from build123d import *

# Parameters (mm, degrees)
SKETCH1_R                                        = 2
BOSS_EXTRUDE1_DEPTH                              = 15
CUT_EXTRUDE7_START                               = 15
SKETCH1_3_R                                      = 5
CUT_EXTRUDE7_DEPTH                               = 4
CUT_EXTRUDE2_START                               = -22.5000001
CUT_EXTRUDE2_DEPTH                               = 45.0000001
CUT_EXTRUDE6_DEPTH                               = 30
CBORE_FOR_M3_HEX_HEAD_MACHINE_SCREW3_D           = 3
CBORE_FOR_M3_HEX_HEAD_MACHINE_SCREW3_DEPTH       = 25
CBORE_FOR_M3_HEX_HEAD_MACHINE_SCREW3_CBORE_D     = 6
CBORE_FOR_M3_HEX_HEAD_MACHINE_SCREW3_CBORE_DEPTH = 18
CBORE_FOR_M3_HEX_HEAD_MACHINE_SCREW3_TIP         = 0.901290929
CUT_EXTRUDE4_START                               = 15
SKETCH19_R                                       = 2.15
SKETCH19_R_2                                     = 2.25
CUT_EXTRUDE4_DEPTH                               = 10
CUT_EXTRUDE5_START                               = -5
SKETCH19_2_R                                     = 2.15
SKETCH19_2_R_2                                   = 2.25
CUT_EXTRUDE5_DEPTH                               = 10
BOSS_EXTRUDE3_DEPTH                              = 2.5
CBORE_FOR_M3_SHCS2_D                             = 3
CBORE_FOR_M3_SHCS2_DEPTH                         = 12
CBORE_FOR_M3_SHCS2_CBORE_D                       = 4.3
CBORE_FOR_M3_SHCS2_CBORE_DEPTH                   = 5.2
CBORE_FOR_M3_SHCS3_D                             = 2.5
CBORE_FOR_M3_SHCS3_DEPTH                         = 12
CBORE_FOR_M3_SHCS3_CBORE_D                       = 4.3
CBORE_FOR_M3_SHCS3_CBORE_DEPTH                   = 5.2
FILLET2_R                                        = 5
CUT_EXTRUDE9_START                               = -15
SKETCH1_5_R                                      = 5
CUT_EXTRUDE9_DEPTH                               = 3


# Read off the part's stored shape, not the designer's step: Cut-Extrude2
with BuildPart() as part:
    # Sketch1 → Boss-Extrude1 (new, symmetric)
    with BuildSketch(Plane.XY):
        with BuildLine():
            Line((0, 17.5), (0, -17.5))
            add(Edge.make_bspline(
                [(0, -17.5), (43.884108447, -9.177006937), (123.842028205, -11.029704256), (170, -22.5)],
                knots=[0, 0, 0, 0, 1, 1, 1, 1], degree=3))
            ThreePointArc((170, -22.5), (192.5, 0), (170, 22.5))
            add(Edge.make_bspline(
                [(170, 22.5), (123.842028205, 11.029704256), (43.884108447, 9.177006937), (0, 17.5)],
                knots=[0.933681919, 0.933681919, 0.933681919, 0.933681919, 1.933681919, 1.933681919, 1.933681919, 1.933681919], degree=3))
        make_face()
        with Locations((175.71763899, 11.115691808)):
            Circle(SKETCH1_R, mode=Mode.SUBTRACT)
        with Locations((164.28236101, -11.115691808)):
            Circle(SKETCH1_R, mode=Mode.SUBTRACT)
        with Locations((178.447925774, -4.345405633)):
            Circle(SKETCH1_R, mode=Mode.SUBTRACT)
        with Locations((161.552074226, 4.345405633)):
            Circle(SKETCH1_R, mode=Mode.SUBTRACT)
    extrude(amount=BOSS_EXTRUDE1_DEPTH, both=True)

    # Sketch1<3> → Cut-Extrude7 (cut)
    with BuildSketch(Plane.XY.offset(CUT_EXTRUDE7_START)):
        with Locations((170, 0)):
            Circle(SKETCH1_3_R)
    extrude(amount=-CUT_EXTRUDE7_DEPTH, mode=Mode.SUBTRACT)

    # Cut-Extrude2 outline → Cut-Extrude2 (cut)
    with BuildSketch(Plane(origin=(0, 0, 0), x_dir=(1, 0, 0), z_dir=(0, 1, 0)).offset(CUT_EXTRUDE2_START)):
        Polygon((14.999999991, -15.000000001), (194, -15), (194, 7.185915493), (192.500000099, 7.000000012), align=None)
    extrude(amount=CUT_EXTRUDE2_DEPTH, mode=Mode.SUBTRACT)

    # Sketch20 → Cut-Extrude6 (cut, symmetric)
    with BuildSketch(Plane(origin=(0, 0, 0), x_dir=(1, 0, 0), z_dir=(0, 1, 0))):
        Polygon((15, -9), (15, 9), (160, 9), (160, 8.971830985), align=None)
    extrude(amount=CUT_EXTRUDE6_DEPTH, both=True, mode=Mode.SUBTRACT)

    # CBORE for M3 Hex Head Machine Screw3
    with Locations(Plane(origin=(0, 0, 10), x_dir=(-1, 0, 0), z_dir=(0, 0, 1))):
        with Locations((-175.71763899, -11.115691808), (-161.552074226, -4.345405633), (-164.28236101, 11.115691808), (-178.447925774, 4.345405633)):
            CounterBoreHole(CBORE_FOR_M3_HEX_HEAD_MACHINE_SCREW3_D / 2, CBORE_FOR_M3_HEX_HEAD_MACHINE_SCREW3_CBORE_D / 2, CBORE_FOR_M3_HEX_HEAD_MACHINE_SCREW3_CBORE_DEPTH, depth=CBORE_FOR_M3_HEX_HEAD_MACHINE_SCREW3_DEPTH)
            with Locations((0, 0, -(CBORE_FOR_M3_HEX_HEAD_MACHINE_SCREW3_DEPTH + CBORE_FOR_M3_HEX_HEAD_MACHINE_SCREW3_TIP / 2))):  # 118° drill point
                Cone(0, CBORE_FOR_M3_HEX_HEAD_MACHINE_SCREW3_D / 2, CBORE_FOR_M3_HEX_HEAD_MACHINE_SCREW3_TIP, mode=Mode.SUBTRACT)

    # Sketch19 → Cut-Extrude4 (cut)
    with BuildSketch(Plane.XY.offset(CUT_EXTRUDE4_START)):
        with Locations((8, 8)):
            Circle(SKETCH19_R)
        with Locations((8, -8)):
            Circle(SKETCH19_R_2)
    extrude(amount=-CUT_EXTRUDE4_DEPTH, mode=Mode.SUBTRACT)

    # Sketch19<2> → Cut-Extrude5 (cut)
    with BuildSketch(Plane.XY.offset(CUT_EXTRUDE5_START)):
        with Locations((8, 8)):
            Circle(SKETCH19_2_R)
        with Locations((8, -8)):
            Circle(SKETCH19_2_R_2)
    extrude(amount=-CUT_EXTRUDE5_DEPTH, mode=Mode.SUBTRACT)

    # Sketch20<3> → Boss-Extrude3 (add, symmetric)
    with BuildSketch(Plane(origin=(0, 0, 0), x_dir=(1, 0, 0), z_dir=(0, 1, 0))):
        Polygon((15, -9), (15, 9), (160, 9), (160, 8.971830985), align=None)
    extrude(amount=BOSS_EXTRUDE3_DEPTH, both=True)

    # CBORE for M3 SHCS2
    with Locations(Plane.XY.offset(15)):
        with Locations((8, 8), (8, -8)):
            CounterBoreHole(CBORE_FOR_M3_SHCS2_D / 2, CBORE_FOR_M3_SHCS2_CBORE_D / 2, CBORE_FOR_M3_SHCS2_CBORE_DEPTH, depth=CBORE_FOR_M3_SHCS2_DEPTH)

    # CBORE for M3 SHCS3
    with Locations(Plane(origin=(0, 0, -15), x_dir=(-1, 0, 0), z_dir=(0, 0, -1))):
        with Locations((-8, 8), (-8, -8)):
            CounterBoreHole(CBORE_FOR_M3_SHCS3_D / 2, CBORE_FOR_M3_SHCS3_CBORE_D / 2, CBORE_FOR_M3_SHCS3_CBORE_DEPTH, depth=CBORE_FOR_M3_SHCS3_DEPTH)

    # Fillet2
    fillet2_edges = [part.edges().sort_by_distance(p)[0] for p in [
        (0, 17.5, -7.5),
        (0, -17.5, 7.5),
    ]]
    fillet(fillet2_edges, radius=FILLET2_R)

    # Sketch1<5> → Cut-Extrude9 (cut)
    with BuildSketch(Plane.XY.offset(CUT_EXTRUDE9_START)):
        with Locations((170, 0)):
            Circle(SKETCH1_5_R)
    extrude(amount=CUT_EXTRUDE9_DEPTH, mode=Mode.SUBTRACT)


solid = part.part
Check sheet for the modelled part. Datum: model origin and axes. Units: mm. A direction names the side the tool comes from. Round coordinates to 2 decimals unless told otherwise and drop trailing zeros. Put each result on its own line as item: value. Start each with the question number.
1. Gauge pin test, flat ends, axial feed: pin 1 (9 mm diameter, centred on x = 86.5, z = -3.5, fed in from +Y); pin 2 (2.5 mm diameter, centred on x = 8, y = 8, fed in from +Z); pin 3 (1 mm diameter, centred on x = 68.5, z = -5, fed in from -Y). Record the tip position at first contact, or that the pin passes through.
2. Draft check along Y on faces 5 (the face through (72, -2.5, -2)), 6 (the face through (104.992, -0.315, 3.846)), 7 (the face through (9.16, 9.81, -9.93)). Enter one of: +Y half, -Y half, draft (parallel to the pull), parting line (faces both ways), or undercut.
3. Section check A-A (z = 7). Give the number of separate pieces and of enclosed holes in the cut face, plus the area to 3 significant figures.
4. Access from +Z, -Z, +X, -X, +Y, -Y to the whole of each face (thin tool, end or side, straight path). Record for faces 1 (the face through (158.69, 3.44, -5.36)), 2 (the face through (9, -9, -5)), 3 (the face through (15, 9, 0)), 4 (the face through (15, -9, 0)).
5. Scan lines: probe 1 along Y at (x, z) = (8, 4.4); probe 2 along Y at (x, z) = (17.5, 0); probe 3 along Y at (x, z) = (8, -7). Record each from-to range of solid material in increasing order.
Findings:
1. pin 1: stops at y = 12.75
1. pin 2: stops at z = 3
1. pin 3: stops at y = -2.5
2. face 5: -Y half
2. face 6: draft
2. face 7: undercut
3. separate pieces: 1
3. enclosed holes: 2
3. area: 1,750 mm^2
4. face 1: +Z
4. face 2: -Z
4. face 3: +Y
4. face 4: -Y
5. probe 1: y = -16.15 to -9.5, -6.5 to 6.5, 9.5 to 16.15
5. probe 2: y = -2.5 to 2.5
5. probe 3: y = -16.15 to -10.25, -5.75 to 5.85, 10.15 to 16.15
